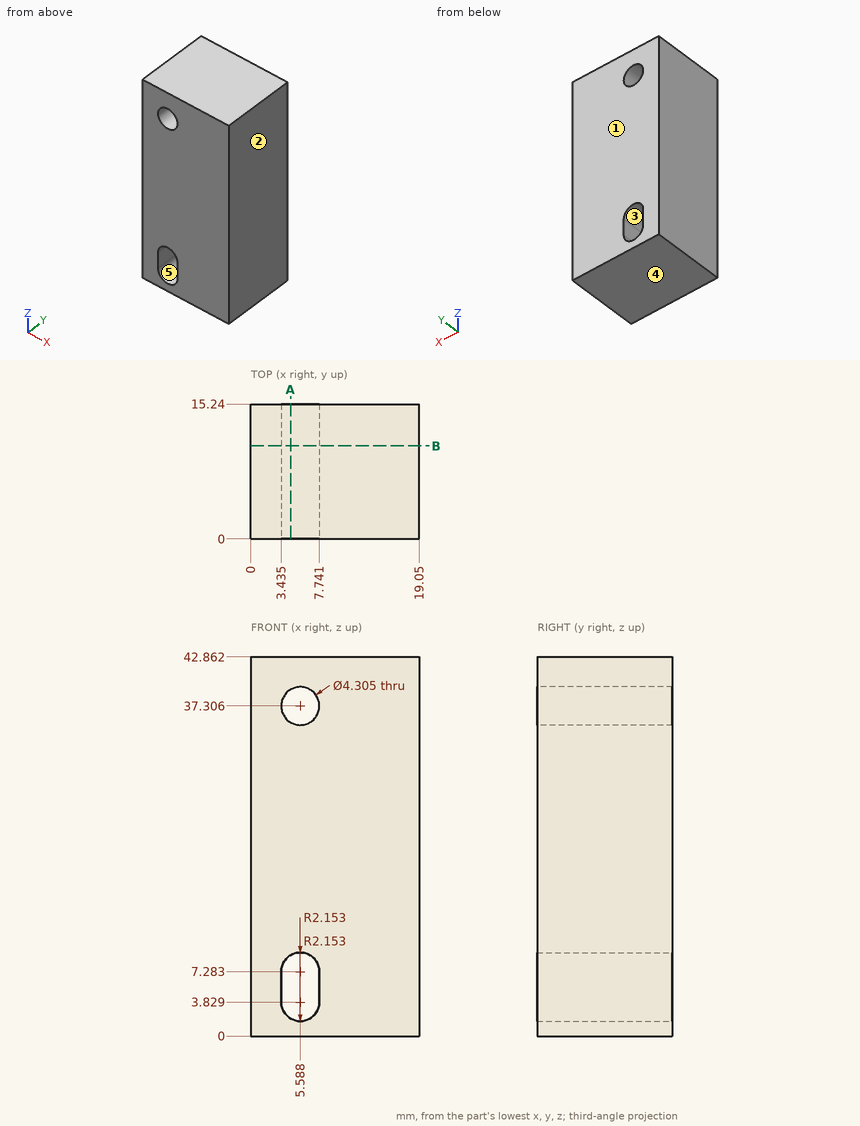
Geometry: see drawing. Coordinates: mm, zero at the bounding-box minimum. A direction names the side the tool comes from. Coordinates: 2 decimals unless noted, no trailing zeros. Write each loop counter-clockwise with the first axis right and the second up, starting at its lowest first coordinate (ties: lowest second). Pieces come first, ordered by that corner, then holes.
1) Mould query, pull axis X, two halves, no side actions, for the marked faces 1, 2 and 3. Classes: pulls with the +X half, pulls with the -X half, needs draft (parallel to the pull), parting line crosses it, or undercut.
2) Section A-A on x = 4.5. Output: boundary loops of the cut face in (y, z).
3) Material intervals for line 1 along Z through (x, y) = (5.75, 12.25); line 2 along Z through (x, y) = (6.5, 9.5) (1 decimal); line 3 along X through (y, z) = (7, 8), sorted ascending.
4) Set-up query: the marked faces 4 and 5. Return all of +Z, -Z, +X, -X, +Y, -Y with unobstructed straight access to the full face (end or side cutting, diameter ignored); none if empty.
5) Section B-B on y = 10.5. State how many separate pieces and enclosed holes the cut face has.
Check result:
1. face 1: needs draft
1. face 2: pulls with the +X half
1. face 3: undercut
2. outline: (0, 0) - (15.24, 0) - (15.24, 1.97) - (0, 1.97) - close; (0, 9.14) - (15.24, 9.14) - (15.24, 35.45) - (0, 35.45) - close; (0, 39.16) - (15.24, 39.16) - (15.24, 42.86) - (0, 42.86) - close
3. line 1: z = 0 to 1.68, 9.43 to 35.16, 39.45 to 42.86
3. line 2: z = 0 to 1.9, 9.2 to 35.4, 39.3 to 42.9
3. line 3: x = 0 to 3.56, 7.62 to 19.05
4. face 4: -Z, +X, -X, +Y, -Y
4. face 5: +Y, -Y
5. separate pieces: 1
5. enclosed holes: 2
